Autodesk Inventor part; units mm, degrees
ref_plane "YZ Plane" through (0, 0, 0) normal (1, 0, 0) x (0, 1, 0)
ref_plane "XZ Plane" through (0, 0, 0) normal (0, 1, 0) x (-1, 0, 0)
ref_plane "XY Plane" through (0, 0, 0) normal (0, 0, 1) x (1, 0, 0)
sketch "スケッチ1" plane through (0, 0, 0) normal (0, 1, 0) x (-1, 0, 0)
  line L0 (-21, 51.2893) -> (-21, -42)
  line L1 (-21, -42) -> (21, -42)
  line L2 (21, -42) -> (21, 51.2893)
  line L3 (-21, 51.2893) -> (21, 51.2893)
  line L4 (-19.7, 0.7) -> (19.7, 0.7)
  line L5 (19.7, 0.7) -> (19.7, -28.3561)
  arc A0 (8.8769, -40.7) -> (19.7, -28.3561) centre (0, -22) ccw
  line L6 (8.8769, -40.7) -> (-8.8769, -40.7)
  arc A1 (-19.7, -28.3561) -> (-8.8769, -40.7) centre (0, -22) ccw
  line L7 (-19.7, -28.3561) -> (-19.7, 0.7)
  line L8 (-19.7, 2.3) -> (-19.7, 33.1604)
  ellipse E0 centre (-12, 33.1604) end of major axis (-12, 25.3416) minor radius 7.7 (-19.3049, 35.6329) -> (-19.7, 33.1604) ccw
  line L9 (-16.2595, 44.9098) -> (-19.3049, 35.6329)
  ellipse E1 centre (-8.9547, 42.4373) end of major axis (-8.9547, 34.6185) minor radius 7.7 (-8.9547, 50.2561) -> (-16.2595, 44.9098) ccw
  line L10 (8.9547, 50.2561) -> (-8.9547, 50.2561)
  ellipse E2 centre (8.9547, 42.4373) end of major axis (8.9547, 34.6185) minor radius 7.7 (16.2595, 44.9098) -> (8.9547, 50.2561) ccw
  line L11 (19.3049, 35.6329) -> (16.2595, 44.9098)
  ellipse E3 centre (12, 33.1604) end of major axis (12, 25.3416) minor radius 7.7 (19.7, 33.1604) -> (19.3049, 35.6329) ccw
  line L12 (19.7, 33.1604) -> (19.7, 2.3)
  line L13 (19.7, 2.3) -> (-19.7, 2.3)
  line L14 (8.9547, 49.6561) -> (-8.9547, 49.6561)
  line L15 (-15.6895, 44.7227) -> (-18.7348, 35.4458)
  line L16 (-19.1, 33.1604) -> (-19.1, 2.9)
  line L17 (-19.1, 2.9) -> (19.1, 2.9)
  line L18 (19.1, 2.9) -> (19.1, 33.1604)
  line L19 (18.7348, 35.4458) -> (15.6895, 44.7227)
  line L20 (19.1, -28.261) -> (19.1, 0.1)
  line L21 (19.1, 0.1) -> (-19.1, 0.1)
  line L22 (-19.1, 0.1) -> (-19.1, -28.261)
  arc A2 (-19.1, -28.261) -> (-8.7407, -40.1) centre (0, -22) ccw
  line L23 (-8.7407, -40.1) -> (8.7407, -40.1)
  arc A3 (8.7407, -40.1) -> (19.1, -28.261) centre (0, -22) ccw
  line L24 (19.1, 27.3) -> (-19.1, 27.3)
  point P0 (0, 0)
  dimension "d0" = 0.6
  dimension "d1" = 0.6
  dimension "d2" = 25
extrude "押し出し1" add sketch "スケッチ1" against normal blind 6 contours L24 L18 L17 L16 | A3 L23 A2 L22 L21 L20
sketch "スケッチ2" plane through (0, 0, 0) normal (0, 1, 0) x (1, 0, 0)
  line L0 (21, -51.2893) -> (21, 42)
  line L1 (21, 42) -> (-21, 42)
  line L2 (-21, 42) -> (-21, -51.2893)
  line L3 (21, -51.2893) -> (-21, -51.2893)
  line L4 (19.7, -0.7) -> (-19.7, -0.7)
  line L5 (-19.7, -0.7) -> (-19.7, 28.3561)
  arc A0 (-8.8769, 40.7) -> (-19.7, 28.3561) centre (0, 22) ccw
  line L6 (-8.8769, 40.7) -> (8.8769, 40.7)
  arc A1 (19.7, 28.3561) -> (8.8769, 40.7) centre (0, 22) ccw
  line L7 (19.7, 28.3561) -> (19.7, -0.7)
  line L8 (19.7, -2.3) -> (19.7, -33.1604)
  ellipse E0 centre (12, -33.1604) end of major axis (12, -25.3416) minor radius 7.7 (19.3049, -35.6329) -> (19.7, -33.1604) ccw
  line L9 (16.2595, -44.9098) -> (19.3049, -35.6329)
  ellipse E1 centre (8.9547, -42.4373) end of major axis (8.9547, -34.6185) minor radius 7.7 (8.9547, -50.2561) -> (16.2595, -44.9098) ccw
  line L10 (-8.9547, -50.2561) -> (8.9547, -50.2561)
  ellipse E2 centre (-8.9547, -42.4373) end of major axis (-8.9547, -34.6185) minor radius 7.7 (-16.2595, -44.9098) -> (-8.9547, -50.2561) ccw
  line L11 (-19.3049, -35.6329) -> (-16.2595, -44.9098)
  ellipse E3 centre (-12, -33.1604) end of major axis (-12, -25.3416) minor radius 7.7 (-19.7, -33.1604) -> (-19.3049, -35.6329) ccw
  line L12 (-19.7, -33.1604) -> (-19.7, -2.3)
  line L13 (-19.7, -2.3) -> (19.7, -2.3)
  point P0 (0, 0)
extrude "押し出し2" add sketch "スケッチ2" along normal blind 1 contours L3 L2 L1 L0 | L4 L5 A0 L6 A1 L7 | L8 E0 L9 E1 L10 E2 L11 E3 L12 L13
properties part number "sole_paint_support_base"
For this review, take the finished solid that the model builds, in its own axes (mm). A direction names the side the tool comes from. Give positions to 0.01 mm unless a question says otherwise; leave off trailing zeros. Write each loop counter-clockwise with the first axis right and the second up, starting at its lowest first coordinate (ties: lowest second). Pieces come first, ordered by that corner, then holes. Notation, with made-up numbers: M 2,81.5 L 22,81.5 A23 ccw 22,95.5 Z; hole C 29,54 d8. An arc over 180 degrees is marked long. Answer as CSV lines item,"result".
1. Consider section B-B, the plane x = 6. Write out the cut boundary in (y, z), then the cut area to 3 significant figures.
Findings:
outline,"M -6,-40.1 L 0,-40.1 L 0,-42 L 1,-42 L 1,51.29 L 0,51.29 L 0,27.3 L -6,27.3 L -6,2.9 L 0,2.9 L 0,0.1 L -6,0.1 Z"
area,"481 mm2"
2. Consider section D-D, the plane x = -18. Write out the cut boundary in (y, z), then the cut area to 3 significant figures.
Findings:
outline,"M -6,-30.94 L 0,-30.94 L 0,-42 L 1,-42 L 1,51.29 L 0,51.29 L 0,27.3 L -6,27.3 L -6,2.9 L 0,2.9 L 0,0.1 L -6,0.1 Z"
area,"426 mm2"
3. For pin 1 (1.8 mm diameter, centred on y = -3.5, z = -18.5, fed in from -X); pin 2 (1 mm diameter, centred on x = -12.5, y = -4, fed in from -Z); pin 3 (1.8 mm diameter, centred on x = -8.5, y = -1.5, fed in from +Z), all flat-tipped, find the tip position at first contact; note any pin that passes through.
Findings:
pin 1,"stops at x = -19.1"
pin 2,"stops at z = -38.12"
pin 3,"stops at z = 27.3"
4. Draft analysis for pull direction Z (two halves, no side actions). For faces 1 (the flat face through (0, -3, -40.1)), 2 (the flat face through (0, -3, 0.1)), 3 (the flat face through (-19.1, -3, -14)), state which applies: +Z half, -Z half, draft (parallel to the pull), parting line (faces both ways), or undercut.
Findings:
face 1,"-Z half"
face 2,"undercut"
face 3,"draft"
5. For faces 4 (the flat face through (0, -3, 27.3)), 5 (the cylindrical face through (15.2, -2.96, -35.15)), 6 (the flat face through (19.1, -3, -14)), list the 3-axis set-ups (+Z, -Z, +X, -X, +Y, -Y) from which the entire face can be reached by the end or side of a thin tool; tool diameter is ignored.
Findings:
face 4,"+Z, +X, -X, -Y"
face 5,"-Z, +X, -Y"
face 6,"+Z, -Z, +X, -Y"
6. Wall thickness on line 1 (Z direction, x = -8, y = -1.5); line 2 (Y direction, x = 14.5, z = 46); line 3 (X direction, y = -5, z = -18.5): over which ranges is each line inside the solid? List them lowest first.
Findings:
line 1,"z = -40.1 to 0.1, 2.9 to 27.3"
line 2,"y = 0 to 1"
line 3,"x = -19.1 to 19.1"
7. Consider section C-C, the plane z = -8.5. Write out the cut boundary in (x, y).
Findings:
outline,"M -21,0 L -19.1,0 L -19.1,-6 L 19.1,-6 L 19.1,0 L 21,0 L 21,1 L -21,1 Z"
8. Consider section A-A, the plane y = -1.5. Write out the cut boundary in (x, z), then the cut area to 3 significant figures.
Findings:
outline,"M -19.1,-28.26 A20.1 ccw -8.74,-40.1 L 8.74,-40.1 A20.1 ccw 19.1,-28.26 L 19.1,0.1 L -19.1,0.1 Z; M -19.1,2.9 L 19.1,2.9 L 19.1,27.3 L -19.1,27.3 Z"
area,"2,380 mm2"
